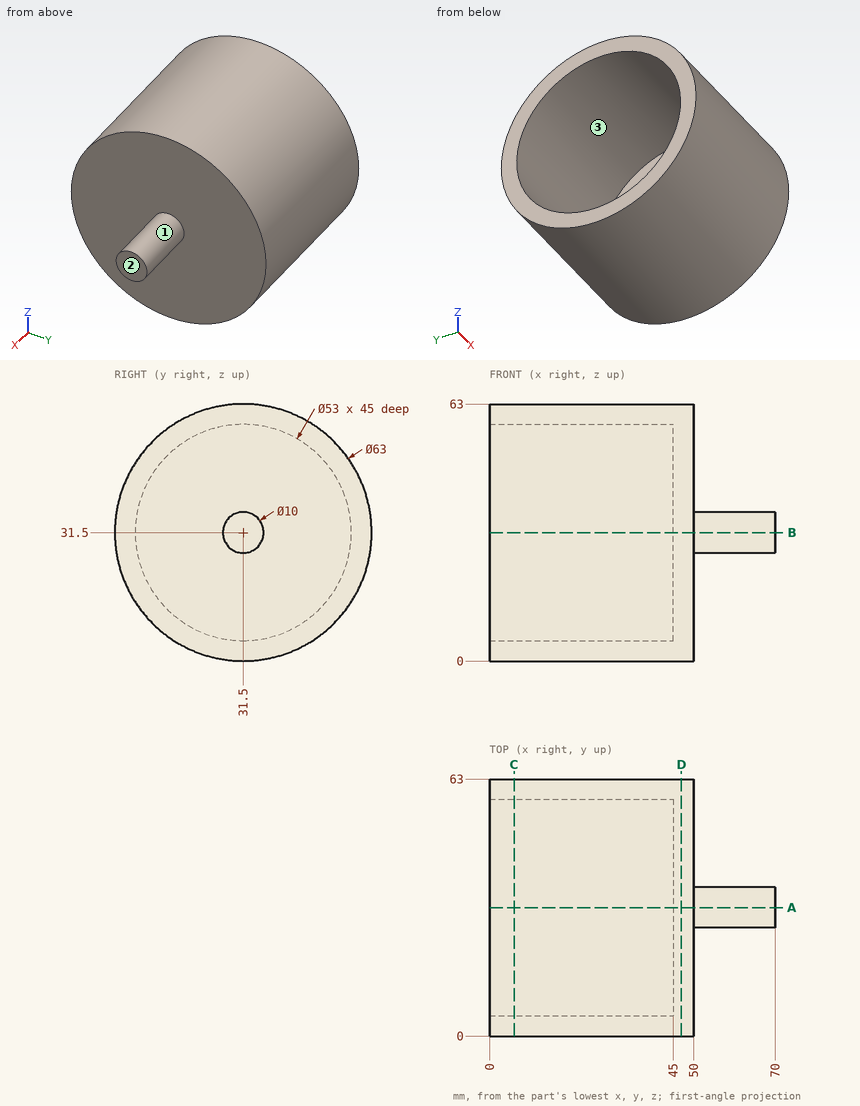
Source: three-view drawing plus pictorial views. Frame: mm from the lowest corner of the part. Round coordinates to 2 decimals unless told otherwise and drop trailing zeros. Write each loop counter-clockwise with the first axis right and the second up, starting at its lowest first coordinate (ties: lowest second). Pieces come first, ordered by that corner, then holes. Notation, with made-up numbers: M -29.5,48 L -19.5,48 A15 ccw -19.5,60 Z; hole C 68,61 d7. An arc over 180 degrees is marked long. Write each question's results on one line, items separated by ' | '.
Q1. Section query D-D (x = 47). Return loops of the section in (y, z), and give its area (3 significant figures).
Results:
outline: C 31.5,31.5 d63 | area: 3,120 mm^2
Q2. Line query: line 1 along Z through (x, y) = (19, 31); line 2 along X through (y, z) = (60, 40). Output: solid intervals per line, ascending.
Results:
line 1: z = 0 to 5, 58 to 63 | line 2: x = 0 to 50
Q3. Section query A-A (y = 31.5). Return loops of the section in (x, z), and give its area (3 significant figures).
Results:
outline: M 0,0 L 50,0 L 50,26.5 L 70,26.5 L 70,36.5 L 50,36.5 L 50,63 L 0,63 L 0,58 L 45,58 L 45,5 L 0,5 Z | area: 965 mm^2
Q4. Section query C-C (x = 6). Return loops of the section in (y, z).
Results:
outline: C 31.5,31.5 d63; hole C 31.5,31.5 d53
Q5. Draft query along Z for the marked faces 1, 2 and 3. Return one class per face: released by +Z, released by -Z, zero draft, split by the parting line, or undercut.
Results:
face 1: split by the parting line | face 2: zero draft | face 3: undercut
Q6. Pin query (flat end, axial travel): P1, Ø2, axis at y = 50.5, z = 41, coming from the +X side; P2, Ø1.5, axis at x = 34.5, y = 10.5, coming from the -Z side; P3, Ø1.5, axis at x = 42.5, z = 7.5, coming from the -Y side. Return the tip coordinate at first contact, or that it passes through.
Results:
P1: stops at x = 50 | P2: stops at z = 7.37 | P3: stops at y = 10.25
